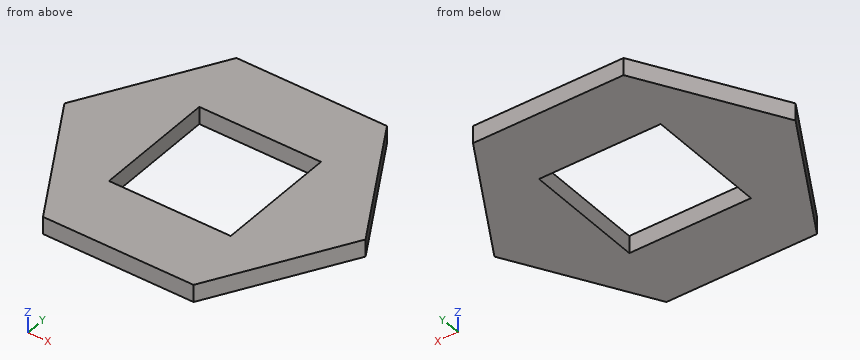
from build123d import *

# Parameters (mm, degrees)
CAP_DEPTH            = 10
SKETCH2_W            = 70
SKETCH2_H            = 70
BATTERY_ACCESS_DEPTH = 116


with BuildPart() as part:
    # Sketch1 → Cap (new body)
    with BuildSketch(Plane.XY):
        Polygon((86.602540378, 0), (43.301270189, 75), (-43.301270189, 75), (-86.602540378, 0), (-43.301270189, -75), (43.301270189, -75), align=None)
    extrude(amount=CAP_DEPTH)

    # Sketch2 → Battery Access (cut, through all)
    with BuildSketch(Plane.XY.offset(10)):
        Rectangle(SKETCH2_W, SKETCH2_H)
    extrude(amount=-BATTERY_ACCESS_DEPTH, mode=Mode.SUBTRACT)


solid = part.part
Input: part model. Units: mm. Frame: model coordinates. Give positions to 0.01 mm unless a question says otherwise; leave off trailing zeros. Write each loop counter-clockwise with the first axis right and the second up, starting at its lowest first coordinate (ties: lowest second). Pieces come first, ordered by that corner, then holes.
Q1. Section A-A, the plane y = -23. Output: boundary loops of the cut face in (x, z), plus the area to 3 significant figures.
Q2. First-contact query: P1, Ø3, axis at y = -7, z = 6.5, coming from the +X side; P2, Ø6, axis at y = -8.5, z = 6, coming from the -X side; P3, Ø1, axis at y = -53, z = 3, coming from the -X side. Flat tips, straight axial feed; report the tip coordinate or a pass-through.
Q3. Material intervals for probe 1 along Y at (x, z) = (-28.5, 5.5); probe 2 along X at (y, z) = (1, 7.75); probe 3 along X at (y, z) = (2.5, 6.5), sorted ascending.
Q4. Section B-B, the plane x = -26. Output: boundary loops of the cut face in (y, z).
Q5. Section D-D, the plane x = -74. Output: boundary loops of the cut face in (y, z), plus the area to 3 significant figures.
Q6. Section C-C, the plane z = 1.5. Output: boundary loops of the cut face in (x, y).
Filled in:
1. outline: (-73.32, 0) - (-35, 0) - (-35, 10) - (-73.32, 10) - close; (35, 0) - (73.32, 0) - (73.32, 10) - (35, 10) - close
1. area: 766 mm2
2. P1: stops at x = 83.43
2. P2: stops at x = -83.43
2. P3: stops at x = -56.29
3. probe 1: y = -75 to -35, 35 to 75
3. probe 2: x = -86.03 to -35, 35 to 86.03
3. probe 3: x = -85.16 to -35, 35 to 85.16
4. outline: (-75, 0) - (-35, 0) - (-35, 10) - (-75, 10) - close; (35, 0) - (75, 0) - (75, 10) - (35, 10) - close
5. outline: (-21.83, 0) - (21.83, 0) - (21.83, 10) - (-21.83, 10) - close
5. area: 437 mm2
6. outline: (-86.6, 0) - (-43.3, -75) - (43.3, -75) - (86.6, 0) - (43.3, 75) - (-43.3, 75) - close; hole (-35, -35) - (35, -35) - (35, 35) - (-35, 35) - close
